Design review of the part shown in the three views and the two pictorial views. Dimensions are in mm from the part's minimum x, y and z. Coordinates: 2 decimals unless noted, no trailing zeros. Write each loop counter-clockwise with the first axis right and the second up, starting at its lowest first coordinate (ties: lowest second). Pieces come first, ordered by that corner, then holes. Notation, with made-up numbers: (4, 4.25) -> (49, 4.25) arc R32 cw to (49, 43.25) -> close; hole circle Ø9 at (10, -34). An arc over 180 degrees is marked (long way). Write each question's results on one line, items separated by ' | '.
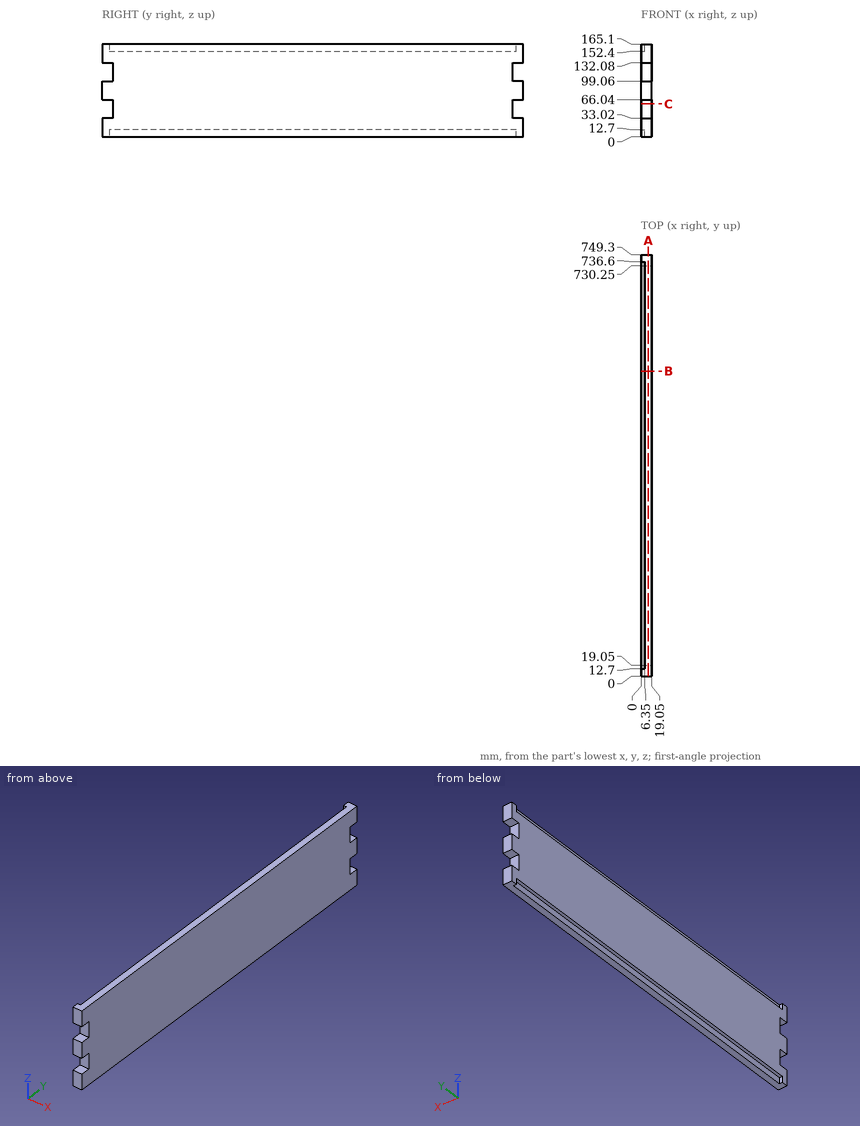
Q1. Clearance check with flat-ended pins moving along their axes: P1, Ø9.5, axis at x = 12, z = 47.5, coming from the +Y side; P2, Ø6.5, axis at y = 236.5, z = 158, coming from the -X side; P3, Ø3, axis at x = 10, z = 108, coming from the -Y side. State where each tip first meets the part, or that it passes through.
Solution:
P1: y = 730.25 | P2: x = 6.35 | P3: y = 19.05
Q2. Add section B-B (y = 542.5). Write out the cut boundary in (x, z), plus the area to 3 significant figures.
Solution:
outline: (0, 12.7) -> (6.35, 12.7) -> (6.35, 0) -> (19.05, 0) -> (19.05, 165.1) -> (6.35, 165.1) -> (6.35, 152.4) -> (0, 152.4) -> close | area: 2,980 mm²
Q3. Add section C-C (z = 58.5). Write out the cut boundary in (x, y).
Solution:
outline: (0, 19.05) -> (19.05, 19.05) -> (19.05, 730.25) -> (0, 730.25) -> close
Q4. Add section A-A (x = 12.75). Write out the cut boundary in (y, z), plus the area to 3 significant figures.
Solution:
outline: (0, 0) -> (749.3, 0) -> (749.3, 33.02) -> (730.25, 33.02) -> (730.25, 66.04) -> (749.3, 66.04) -> (749.3, 99.06) -> (730.25, 99.06) -> (730.25, 132.08) -> (749.3, 132.08) -> (749.3, 165.1) -> (0, 165.1) -> (0, 132.08) -> (19.05, 132.08) -> (19.05, 99.06) -> (0, 99.06) -> (0, 66.04) -> (19.05, 66.04) -> (19.05, 33.02) -> (0, 33.02) -> close | area: 121,000 mm²
Q5. For line 1 (Y direction, x = 2, z = 155); line 2 (X direction, y = 310.5, z = 11.5); line 3 (Y direction, x = 12.25, z = 64), list the stretches that pass through material, from the lowest coordinate up. Write a range as from..to.
Solution:
line 1: 0..12.7, 736.6..749.3 | line 2: 6.35..19.05 | line 3: 19.05..730.25
